Study the drawing (mm; zero at the part's minimum x, y, z) and answer. A direction names the side the tool comes from. Give positions to 0.01 mm unless a question says otherwise; leave off trailing zeros. Write each loop counter-clockwise with the first axis right and the second up, starting at its lowest first coordinate (ties: lowest second). Pieces come first, ordered by that corner, then holes. Notation, with made-up numbers: (-27.75, 87.25) - (-16.75, 87.25) arc R26 ccw to (-16.75, 109.25) - close; hole circle Ø3 at (-12, -25.75). An arc over 180 degrees is marked (long way). Write each question's results on one line, items separated by ' | '. Start each with the question number.
Q1. Find the intervals of material crossed by probe 1 along Y at (x, z) = (43.5, 4); probe 2 along Y at (x, z) = (8.5, 2); probe 3 along Y at (x, z) = (5, 2), in increasing order.
Q2. Flat-ended cylindrical pins translate along their axes: pin 1 Ø1.9 at (x, z) = (38.5, 4.5) entering from -Y; pin 2 Ø3 at (x, z) = (36.5, 5.5) entering from +Y; pin 3 Ø3 at (y, z) = (4, 4.5) entering from +X. Find the tip coordinate at first contact, or state that the pin passes through.
Q3. Section A-A (x = 22) is taken. Determine the outline of the cut face in (y, z).
Q4. For the marked faces 5, 6 and 7, determine the directions among +Z, -Z, +X, -X, +Y, -Y from which every point of the face is accessible in a straight line to the end or side of a thin tool.
Q5. For a pull along Y with two mould halves and no side action, classify the marked faces 1, 2, 3 and 4 as pulls with the +Y half, pulls with the -Y half, needs draft (parallel to the pull), parting line crosses it, or undercut.
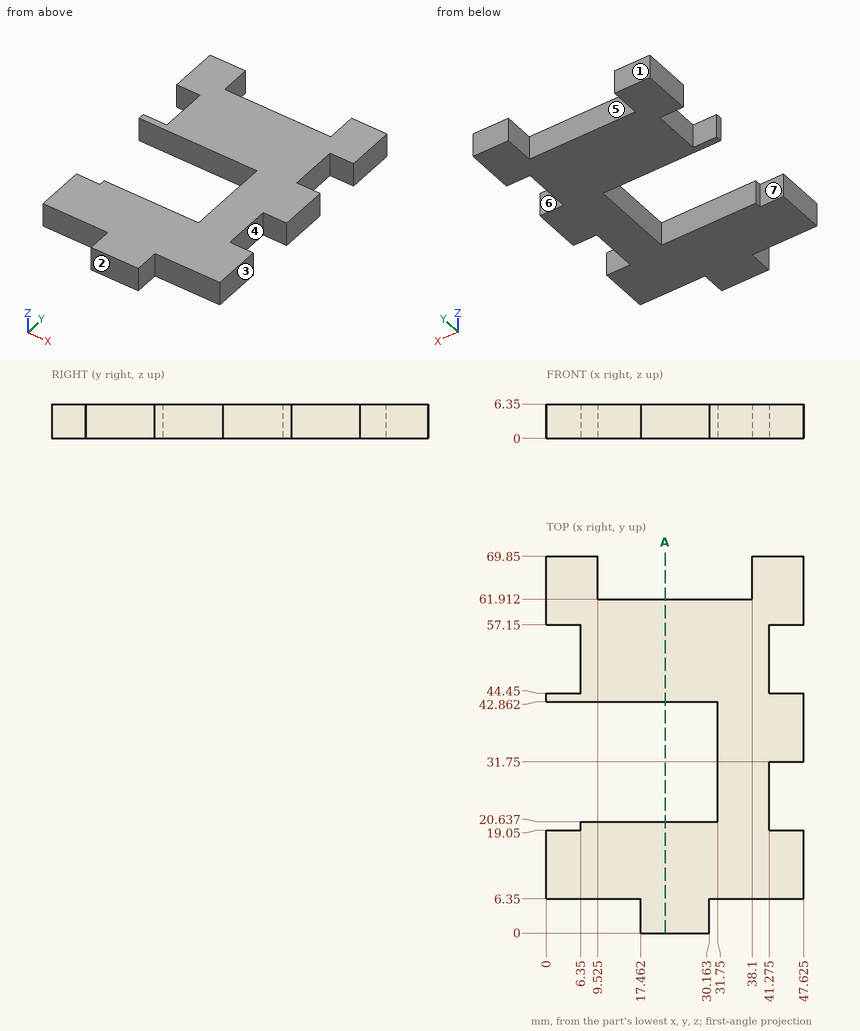
Answers below:
1) probe 1: y = 6.35 to 19.05, 31.75 to 44.45, 57.15 to 69.85 | probe 2: y = 6.35 to 20.64, 42.86 to 69.85 | probe 3: y = 6.35 to 19.05, 42.86 to 44.45, 57.15 to 69.85
2) pin 1: stops at y = 6.35 | pin 2: stops at y = 61.91 | pin 3: stops at x = 30.16
3) outline: (0, 0) - (20.64, 0) - (20.64, 6.35) - (0, 6.35) - close; (42.86, 0) - (61.91, 0) - (61.91, 6.35) - (42.86, 6.35) - close
4) face 5: +Z, -Z, +Y | face 6: +Z, -Z, +X | face 7: +Z, -Z, -X
5) face 1: pulls with the +Y half | face 2: pulls with the -Y half | face 3: needs draft | face 4: undercut
